Geometry check sheet. Reference: the model listing, model coordinates, mm. Round coordinates to 2 decimals unless told otherwise and drop trailing zeros. Write each loop counter-clockwise with the first axis right and the second up, starting at its lowest first coordinate (ties: lowest second). Pieces come first, ordered by that corner, then holes. Notation, with made-up numbers: (40, 48.25) - (46, 48.25) arc R36 cw to (46, 84.25) - close; hole circle Ø2 at (31, 83.25). An arc over 180 degrees is marked (long way). One line per question, with ' | ' between items. Start each with the question number.
Autodesk Inventor part; units mm, degrees
ref_plane "YZ Plane" through (0, 0, 0) normal (1, 0, 0) x (0, 1, 0)
ref_plane "XZ Plane" through (0, 0, 0) normal (0, 1, 0) x (-1, 0, 0)
ref_plane "XY Plane" through (0, 0, 0) normal (0, 0, 1) x (1, 0, 0)
sketch "Sketch1" plane through (0, 0, 0) normal (0, 0, 1) x (1, 0, 0)
  circle A0 centre (0, 0) radius 8
  line L0 (0, 0) -> (0, -24.7) construction
  line L1 (0, -24.7) -> (-19.9, -24.7)
  line L2 (-19.9, -24.7) -> (-19.9, -19.7)
  line L3 (-19.9, -19.7) -> (-9.1, -19.7)
  line L4 (-9.1, -19.7) -> (-3.85, -7.0127)
  line L5 (0, -24.7) -> (19.9, -24.7)
  line L6 (19.9, -24.7) -> (19.9, -19.7)
  line L7 (19.9, -19.7) -> (9.1, -19.7)
  line L8 (9.1, -19.7) -> (3.85, -7.0127)
  line L9 (0, 0) -> (0, 8) construction
  line L10 (-3.85, -7.0127) -> (3.85, -7.0127) construction
  line L11 (-8.85, -24.7) -> (-4.5, -19.1)
  line L12 (-4.5, -19.1) -> (0, -19.1)
  line L13 (0, -19.1) -> (4.5, -19.1)
  line L14 (4.5, -19.1) -> (8.85, -24.7)
  dimension "d0" = 16
  dimension "d1" = 39.8
  dimension "d2" = 5
  dimension "d4" = 10.8
  dimension "d7" = 32.7
  dimension "d8" = 7.7
  dimension "d9" = 9
  dimension "d10" = 5.6
  dimension "d11" = 17.7
extrude "Extrusion1" add sketch "Sketch1" along normal blind 1000 contours A0 | A0 L8 L7 L6 L5 L14 L13 L12 L11 L1 L2 L3 L4
sketch "Sketch2" plane through (-19.9, -19.7, 1000) normal (0, 1, 0) x (1, 0, 0)
  circle A0 centre (5.4, 950) radius 3
  line L0 (10.8, 1000) -> (0, 1000)
  line L1 (5.4, 1000) -> (5.4, 950) construction
  line L2 (0, 1000) -> (11.05, 1000) construction
  point P0 (19.9, 1000)
  dimension "d14" = 50
  dimension "d15" = 6
extrude "Extrusion2" cut sketch "Sketch2" against normal through all
pattern_linear "Rectangular Pattern1" count 7 spacing 150 along (0, 0, 1) of "Extrusion2"
mirror "Mirror1" about plane through (0, 0, 0) normal (1, 0, 0) of "Rectangular Pattern1", "Extrusion2"
properties part number "Linear Rail"
Q1. Section check B-B, the plane y = -13. Record the cut outline in (x, z).
Q2. Thickness scan on line 1 (X direction, y = -23.6, z = 650); line 2 (X direction, y = -22, z = 350); line 3 (X direction, y = -1, z = 111). Record the ranges inside material, lowest first.
Q3. Draft check along Y on faces 1 (the cylindrical face through (0, 8, 493)), 2 (the flat face through (0, -8, 1000)). Enter one of: pulls with the +Y half, pulls with the -Y half, needs draft (parallel to the pull), parting line crosses it, or undercut.
Q4. Section check A-A, the plane z = 94.5. Record the cut outline in (x, y), then the cut area to 3 significant figures.
Q5. Go/stop test with flat-tipped pins: P1, Ø9.5, axis at x = -14.5, z = 350, coming from the +Y side; P2, Ø8, axis at y = -15, z = 506, coming from the +X side; P3, Ø3.5, axis at x = -14.5, z = 800, coming from the -Y side; P4, Ø10, axis at y = 2.5, z = 555, coming from the -X side. Record where each tip stops, or that it passes through.
Result sheet:
1) outline: (-6.33, 0) - (6.33, 0) - (6.33, 1000) - (-6.33, 1000) - close
2) line 1: -19.9 to -17.5, -11.5 to -8, 8 to 11.5, 17.5 to 19.9 | line 2: -19.9 to -17.5, -11.5 to -6.75, 6.75 to 11.5, 17.5 to 19.9 | line 3: -7.94 to 7.94
3) face 1: undercut | face 2: needs draft
4) outline: (-19.9, -24.7) - (-8.85, -24.7) - (-4.5, -19.1) - (4.5, -19.1) - (8.85, -24.7) - (19.9, -24.7) - (19.9, -19.7) - (9.1, -19.7) - (3.85, -7.01) arc R8 ccw (long way) to (-3.85, -7.01) - (-9.1, -19.7) - (-19.9, -19.7) - close | area: 484 mm²
5) P1: y = -19.7 | P2: x = 8.81 | P3: through | P4: x = -8
